The model under review builds one solid part; all positions refer to its coordinate system, in mm. Face numbers are marked on the shaded views. A direction names the side the tool comes from. Give positions to 0.01 mm unless a question says otherwise; leave off trailing zeros. Write each loop counter-clockwise with the first axis right and the second up, starting at its lowest first coordinate (ties: lowest second). Pieces come first, ordered by that corner, then holes. Notation, with made-up numbers: (74, 34) - (94, 34) arc R26 cw to (94, 54) - close; hole circle Ø9 at (28.25, 4). An arc over 180 degrees is marked (long way). One line per question, with ' | ' between items. Start each with the question number.
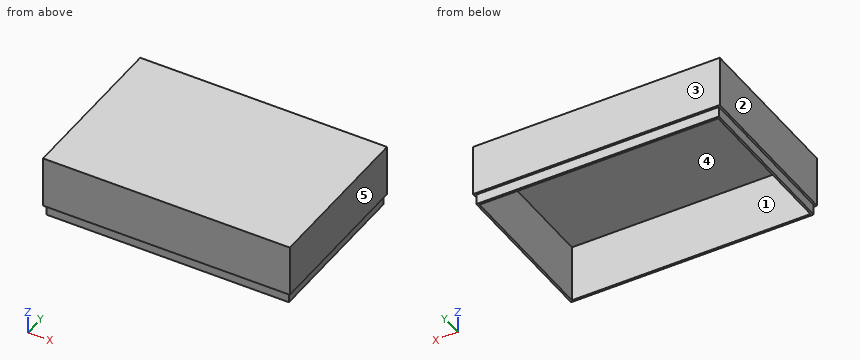
```python
from build123d import *

# Parameters (mm, degrees)
SKETCH1_W           = 120
SKETCH1_H           = 80
BOSS_EXTRUDE1_DEPTH = 30
SHELL1_T            = -2
SKETCH10_W          = 120
SKETCH10_H          = 80
SKETCH10_W_2        = 118
SKETCH10_H_2        = 78
CUT_EXTRUDE1_DEPTH  = 5


with BuildPart() as part:
    # Sketch1 → Boss-Extrude1 (new body)
    with BuildSketch(Plane.XY):
        Rectangle(SKETCH1_W, SKETCH1_H)
    extrude(amount=BOSS_EXTRUDE1_DEPTH)

    # Shell1
    shell1_openings = [part.faces().sort_by_distance(p)[0] for p in [
        (0, 0, 0),
    ]]
    offset(amount=SHELL1_T, openings=shell1_openings, kind=Kind.INTERSECTION)

    # Sketch10 → Cut-Extrude1 (cut)
    with BuildSketch(Plane(origin=(0, 0, 0), x_dir=(-1, 0, 0), z_dir=(0, 0, -1))):
        Rectangle(SKETCH10_W, SKETCH10_H)
        Rectangle(SKETCH10_W_2, SKETCH10_H_2, mode=Mode.SUBTRACT)
    extrude(amount=-CUT_EXTRUDE1_DEPTH, mode=Mode.SUBTRACT)


solid = part.part
```
Item 1: Take a section at C-C (x = 50). Give the boundary of the cut face in (y, z), plus the area to 3 significant figures.
Item 2: The part is to be moulded in two halves that separate along X. For the marked faces 3, 4 and 5, say which applies: +X half, -X half, draft (parallel to the pull), parting line (faces both ways), or undercut.
Item 3: Take a section at A-A (z = 18.5). Give the boundary of the cut face in (x, y).
Item 4: Clearance check with flat-ended pins moving along their axes: P1, Ø10, axis at x = -38.5, y = -22, coming from the -Z side; P2, Ø2.5, axis at x = -4, z = 2.5, coming from the -Y side; P3, Ø4, axis at x = -16, z = 2.5, coming from the +Y side. State where each tip first meets the part, or that it passes through.
Item 5: Take a section at B-B (y = -2.5). Give the boundary of the cut face in (x, z).
Item 6: For probe 1 along X at (y, z) = (3, 6); probe 2 along Y at (x, z) = (-22, 3.75); probe 3 along X at (y, z) = (26, 3.75), list the stretches that pass through material, from the lowest coordinate up.
Item 7: Machinability: for the marked faces 1 and 2, which of the approach directions +Z, -Z, +X, -X, +Y, -Y give a long, thin tool a straight path to every point of the face, cutting with its end or side? Answer none if there is none.
Check sheet entries:
1) outline: (-40, 5) - (-39, 5) - (-39, 0) - (-38, 0) - (-38, 28) - (38, 28) - (38, 0) - (39, 0) - (39, 5) - (40, 5) - (40, 30) - (-40, 30) - close | area: 262 mm^2
2) face 3: draft | face 4: undercut | face 5: +X half
3) outline: (-60, -40) - (60, -40) - (60, 40) - (-60, 40) - close; hole (-58, -38) - (58, -38) - (58, 38) - (-58, 38) - close
4) P1: stops at z = 28 | P2: stops at y = -39 | P3: stops at y = 39
5) outline: (-60, 5) - (-59, 5) - (-59, 0) - (-58, 0) - (-58, 28) - (58, 28) - (58, 0) - (59, 0) - (59, 5) - (60, 5) - (60, 30) - (-60, 30) - close
6) probe 1: x = -60 to -58, 58 to 60 | probe 2: y = -39 to -38, 38 to 39 | probe 3: x = -59 to -58, 58 to 59
7) face 1: -Z | face 2: +Z, -Z, -X, +Y, -Y
